Autodesk Inventor part; units mm, degrees
ref_plane "YZ Plane" through (0, 0, 0) normal (1, 0, 0) x (0, 1, 0)
ref_plane "XZ Plane" through (0, 0, 0) normal (0, 1, 0) x (-1, 0, 0)
ref_plane "XY Plane" through (0, 0, 0) normal (0, 0, 1) x (1, 0, 0)
sketch "Sketch4" plane through (0, 0, 0) normal (0, 0, 1) x (1, 0, 0)
  line L0 (0, 0) -> (15, 0)
  line L1 (15, 0) -> (0, 7.5)
  line L2 (0, 7.5) -> (0, 0)
  line L3 (0, 5) -> (5, 5)
  dimension "d4" = 15
  dimension "d5" = 7.5
  dimension "d6" = 2.5
revolve "Revolution1" add sketch "Sketch4" angle 360 about axis through (0, 7.5, 0) along (0, -1, 0) contours L2 L3 L1 L0
sketch "Sketch5" plane through (0, 0, 0) normal (0, -1, 0) x (1, 0, 0)
  circle A0 centre (0, 0) radius 15
  point P0 (0, 0)
  dimension "d17" = 30
extrude "Extrusion2" add sketch "Sketch5" along normal blind 210
sketch "Sketch7" plane through (0, 5, 0) normal (0, 1, 0) x (1, 0, 0)
  circle A0 centre (0, 0) radius 5
  point P0 (0, 0)
  dimension "d18" = 10
extrude "Extrusion4" add sketch "Sketch7" along normal blind 10
sketch "Sketch8" plane through (0, 15, 0) normal (0, 1, 0) x (1, 0, 0)
  circle A0 centre (0, 0) radius 7.5
  line L0 (0, -7.5) -> (0, 7.5)
  point P0 (0, 0)
  dimension "d19" = 15
ref_plane "Work Plane1" through (0, 15, 0) normal (0, 0, -1) x (-1, 0, 0)
sketch "Sketch9" plane through (0, 15, 0) normal (0, 0, -1) x (-1, 0, 0)
  line L0 (0, 0) -> (7.5, 0)
  line L1 (0, 0) -> (0, 7.5)
  circle A0 centre (0, 0) radius 7.5
  line L2 (0, 0) -> (-7.5, 0)
  point P0 (0, -15)
  dimension "d20" = 7.5
  dimension "d21" = 7.5
revolve "Revolution2" add sketch "Sketch9" angle 360 about axis through (0, 15, 0) along (0, 1, 0) contours L1 A0 L0
properties part number "Shafts"
Part model, mm, in its own coordinate system. Round coordinates to 2 decimals unless told otherwise and drop trailing zeros. Write each loop counter-clockwise with the first axis right and the second up, starting at its lowest first coordinate (ties: lowest second). Pieces come first, ordered by that corner, then holes. Notation, with made-up numbers: M 12,-3.75 L 60,-3.75 A26 ccw 60,13.25 Z; hole C 42.25,-34.75 d1. An arc over 180 degrees is marked long. Return JSON: item names as keys, results as strings. Group by question number.
(1) Saw through at A-A on z = 0. Write the cut outline in (x, y), then the cut area to 3 significant figures.
(2) Pin check, flat tips, straight feed: pin 1 Ø1 at (x, y) = (3, -174.5) entering from -Z; pin 2 Ø1.5 at (y, z) = (-118, 9) entering from +X; pin 3 Ø4 at (y, z) = (-42, -6) entering from +X. Stop position of each tip, or through.
(3) Drill centre lines: probe 1 along Z at (x, y) = (0.5, -126); probe 2 along Y at (x, z) = (-3.25, 4); probe 3 along X at (y, z) = (-66, -0.25). Where is each one in solid material? Low to high.
(4) Saw through at B-B on x = 0. Write the cut outline in (y, z).
(5) Two-plate mould, pull along Y, no slides. Class faces 1 (the face through (-1.22, 4.69, -5.49)), 2 (the face through (-14.985, -103.53, -0.66)), 3 (the face through (-2, 15, -5)), 4 (the face through (0, -210, 0)): +Y half, -Y half, draft (parallel to the pull), parting line (faces both ways), or undercut.
(6) Saw through at C-C on y = -54. Write the cut outline in (x, z), then the cut area to 3 significant figures.
Returned:
{
 "1": {"outline": "M -15,-210 L 15,-210 L 15,0 L 5,5 L 5,15 L 7.5,15 A7.5 ccw -7.5,15 L -5,15 L -5,5 L -15,0 Z", "area": "6,590 mm²"},
 "2": {"pin 1": "z = -14.79", "pin 2": "x = 12.53", "pin 3": "x = 14.46"},
 "3": {"probe 1": "-14.99 to 14.99", "probe 2": "-210 to 4.92, 15 to 20.45", "probe 3": "-15 to 15"},
 "4": {"outline": "M -210,-15 L 0,-15 L 5,-5 L 15,-5 L 15,-7.5 A7.5 ccw 15,7.5 L 15,5 L 5,5 L 0,15 L -210,15 Z"},
 "5": {"face 1": "undercut", "face 2": "draft", "face 3": "undercut", "face 4": "-Y half"},
 "6": {"outline": "C 0,0 d30", "area": "707 mm²"}
}
